from build123d import *

# Parameters (mm, degrees)
BOSS_EXTRUDE1_DEPTH = 2
SKETCH2_R           = 5.5
SKETCH2_R_2         = 1.5
CUT_EXTRUDE1_DEPTH  = 2


with BuildPart() as part:
    # Sketch1 → Boss-Extrude1 (new body)
    with BuildSketch(Plane(origin=(0, 0, 0), x_dir=(1, 0, 0), z_dir=(0, 1, 0))):
        with BuildLine():
            Line((75, -10), (-75, -10))
            Line((-75, -10), (-75, 10))
            ThreePointArc((-75, 10), (0, 75.663729752), (75, 10))
            Line((75, 10), (75, -10))
        make_face()
        with BuildLine():
            Line((-63.679706635, 16.019374764), (63.679706635, 16.019374764))
            ThreePointArc((63.679706635, 16.019374764), (0, 65.663729752), (-63.679706635, 16.019374764))
        make_face(mode=Mode.SUBTRACT)
    extrude(amount=BOSS_EXTRUDE1_DEPTH)

    # Sketch2 → Cut-Extrude1 (cut)
    with BuildSketch(Plane(origin=(0, 2, 0), x_dir=(1, 0, 0), z_dir=(0, 1, 0))):
        with Locations(Location((0, 0, 0), (0, 0, 270))):
            Circle(SKETCH2_R)
        with Locations(Location((65, 0, 0), (0, 0, 270))):
            Circle(SKETCH2_R_2)
    extrude(amount=-CUT_EXTRUDE1_DEPTH, mode=Mode.SUBTRACT)


solid = part.part
Design review of the part built by this model. Coordinates are the model's own, in mm. Coordinates: 2 decimals unless noted, no trailing zeros. Loops run counter-clockwise (first coordinate to the right, second up) from the corner with the lowest first, then second, coordinate; pieces in that order, holes last. Notation, with made-up numbers: (37, -19.75) - (93, -19.75) arc R26 cw to (93, 2.25) - close; hole circle Ø8 at (3.25, 8.5). An arc over 180 degrees is marked (long way). Use CSV: the item, a comma, the result in double quotes. Start each with the question number.
1. Mouldability with a two-part tool opening along Z and no side actions: class faces 1 (the flat face through (1, 2, -14)), 2 (the cylindrical face through (1.217, 0.986, -65.652)), 3 (the cylindrical face through (-1.52, 0.99, -75.65)) as released by +Z, released by -Z, zero draft, split by the parting line, or undercut.
2. Clearance check with a flat-ended pin moving along its axis: pin 1 (3.5 mm diameter, centred on x = 65, z = 0, fed in from +Y). State where the tip first meets the part, or that it passes through.
3. Add section C-C on y = 1.15. Give the boundary of the cut face in (x, z).
4. Add section D-D on x = -20. Give the boundary of the cut face in (y, z).
5. To check wall thickness, follow probe 1 along X at (y, z) = (1.4, 0); probe 2 along Z at (x, y) = (-1.5, 1.9); probe 3 along Z at (x, y) = (51, 0.4). State the ranges of each line that lie inside material, in increasing order.
6. Add section A-A on x = 0. Give the boundary of the cut face in (y, z), plus the area to 3 significant figures.
7. Add section B-B on z = 0. Give the boundary of the cut face in (x, y).
Resolved:
1,face 1,"zero draft"
1,face 2,"undercut"
1,face 3,"released by -Z"
2,pin 1,"y = 2"
3,outline,"(-75, -10) arc R75.66 ccw to (75, -10) - (75, 10) - (-75, 10) - close; hole (-63.68, -16.02) arc R65.66 ccw to (63.68, -16.02) - close; hole circle Ø11 at (0, 0); hole circle Ø3 at (65, 0)"
4,outline,"(0, -72.97) - (2, -72.97) - (2, -62.54) - (0, -62.54) - close; (0, -16.02) - (2, -16.02) - (2, 10) - (0, 10) - close"
5,probe 1,"-75 to -5.5, 5.5 to 63.5, 66.5 to 75"
5,probe 2,"-75.65 to -65.65, -16.02 to -5.29, 5.29 to 10"
5,probe 3,"-55.89 to -41.36, -16.02 to 10"
6,outline,"(0, -75.66) - (2, -75.66) - (2, -65.66) - (0, -65.66) - close; (0, -16.02) - (2, -16.02) - (2, -5.5) - (0, -5.5) - close; (0, 5.5) - (2, 5.5) - (2, 10) - (0, 10) - close"
6,area,"50.0 mm2"
7,outline,"(-75, 0) - (-5.5, 0) - (-5.5, 2) - (-75, 2) - close; (5.5, 0) - (63.5, 0) - (63.5, 2) - (5.5, 2) - close; (66.5, 0) - (75, 0) - (75, 2) - (66.5, 2) - close"
